Source: CAD feature listing. Evaluate the final solid. Frame: model axes, mm. A direction names the side the tool comes from. Give positions to 0.01 mm unless a question says otherwise; leave off trailing zeros. Order: outer loops, then holes, each group sorted by start corner. A loop starts at its lowest first (then second) coordinate and runs counter-clockwise, first axis right, second up.
Autodesk Inventor part; units mm, degrees
ref_plane "YZ Plane" through (0, 0, 0) normal (1, 0, 0) x (0, 1, 0)
ref_plane "XZ Plane" through (0, 0, 0) normal (0, 1, 0) x (-1, 0, 0)
ref_plane "XY Plane" through (0, 0, 0) normal (0, 0, 1) x (1, 0, 0)
sketch "Sketch1" plane through (0, 0, 0) normal (0, 1, 0) x (-1, 0, 0)
  line L0 (0, 0) -> (-120, 0)
  line L1 (-120, 0) -> (-120, -100)
  line L2 (-120, -100) -> (0, -100)
  line L3 (0, -100) -> (0, 0)
  dimension "d0" = 120
  dimension "d1" = 100
extrude "Extrusion1" add sketch "Sketch1" along normal blind 3
sketch "Sketch2" plane through (0, 3, 0) normal (0, 1, 0) x (1, 0, 0)
  line L0 (0, 100) -> (0, 0) construction
  line L1 (0, 0) -> (3, 0) construction
  line L2 (3, 0) -> (3, 3) construction
  line L3 (3, 3) -> (0, 3) construction
  line L4 (0, 3) -> (0, 0) construction
  line L5 (120, 100) -> (0, 100) construction
  line L6 (120, 100) -> (117, 100) construction
  line L7 (117, 100) -> (117, 97) construction
  line L8 (117, 97) -> (120, 97) construction
  line L9 (120, 97) -> (120, 100) construction
  line L10 (3, 3) -> (117, 3)
  line L11 (117, 3) -> (117, 97)
  line L12 (117, 97) -> (3, 97)
  line L13 (3, 97) -> (3, 3)
  line L14 (120, 0) -> (120, 100)
  line L15 (0, 0) -> (120, 0)
  line L16 (120, 0) -> (120, 100)
  line L17 (120, 100) -> (0, 100)
  line L18 (0, 100) -> (0, 0)
  dimension "d4" = 3
  dimension "d5" = 3
  dimension "d6" = 3
  dimension "d7" = 3
extrude "Extrusion2" add sketch "Sketch2" along normal blind 97
ref_plane "Work Plane1" through (155, 0, 0) normal (1, 0, 0) x (0, 0, -1)
sketch "Sketch3" plane through (155, 0, 0) normal (1, 0, 0) x (0, 0, -1)
  line L0 (0, 0) -> (0, 100) construction
  line L1 (0, 0) -> (50, 0) construction
  line L2 (100, 0) -> (0, 0) construction
  line L3 (50, 0) -> (50, 35) construction
  line L4 (50, 35) -> (43, 35) construction
  line L5 (50, 35) -> (50, 73) construction
  line L6 (50, 73) -> (40, 73) construction
  line L7 (40, 73) -> (40, 54) construction
  line L8 (43, 35) -> (40, 54)
  line L9 (40, 54) -> (40, 73)
  line L10 (3, 100) -> (97, 100) construction
  line L11 (50, 100) -> (15, 100) construction
  line L12 (15, 100) -> (15, 97)
  line L13 (15, 97) -> (40, 73)
  line L14 (15, 100) -> (43, 73)
  line L15 (43, 73) -> (43, 54)
  line L16 (43, 35) -> (45, 35)
  line L17 (43, 54) -> (45, 35)
  dimension "d11" = 35
  dimension "d12" = 7
  dimension "d13" = 38
  dimension "d14" = 10
  dimension "d15" = 35
  dimension "d16" = 3
  dimension "d81" = 19
  dimension "d82" = 3
  dimension "d83" = 2
  dimension "d84" = 19
revolve "Revolution1" add sketch "Sketch3" angle 360 about axis through (155, 35, -50) along (0, 1, 0)
sketch "Sketch4" plane through (0, 100, 0) normal (0, 1, 0) x (1, 0, 0)
  line L0 (120, 0) -> (120, 100)
  line L1 (120, 0) -> (120, 3)
  line L2 (120, 100) -> (0, 100)
  line L3 (120, 100) -> (120, 97)
  line L4 (120, 97) -> (120, 3)
  circle A0 centre (155, 50) radius 5
  circle A1 centre (155, 50) radius 35
  circle A2 centre (155, 50) radius 38
  line L5 (120, 0) -> (120, 100)
  line L6 (120, 0) -> (155, 12)
  line L7 (155, 88) -> (120, 100)
  point P0 (0, 0)
  point P1 (120, 50)
  dimension "d18" = 3
  dimension "d19" = 3
  dimension "d89" = 70
  dimension "d90" = 3
extrude "Extrusion3" add sketch "Sketch4" against normal blind 3 contours L0 A2 L6 | A2 L0 | L0 L7 A2 picked at (191.3899, 55.4147)
sketch "Sketch5" plane through (0, 100, 0) normal (0, 1, 0) x (1, 0, 0)
  line L0 (120, 0) -> (120, 100)
  line L1 (0, 100) -> (0, 0)
  line L2 (120, 0) -> (0, 0)
  line L3 (0, 0) -> (0, 100)
  line L4 (0, 100) -> (120, 100)
  line L5 (120, 100) -> (120, 0)
  circle A0 centre (155, 50) radius 35
  line L6 (117, 3) -> (117, 97)
  line L7 (117, 3) -> (3, 3)
  line L8 (3, 3) -> (3, 97)
  line L9 (117, 3) -> (3, 3)
  line L10 (3, 3) -> (3, 97)
  line L11 (3, 97) -> (117, 97)
  line L12 (117, 97) -> (117, 3)
  circle A1 centre (155, 50) radius 35
  circle A2 centre (155, 50) radius 38
  line L13 (0, 0) -> (120, 0)
  line L14 (120, 100) -> (155, 88)
  line L15 (120, 100) -> (155, 88)
  line L16 (155, 12) -> (120, 0)
  line L17 (120, 0) -> (155, 12)
  line L18 (120, 50) -> (120, 0)
  line L19 (120, 3) -> (155, 15)
  line L20 (120, 100) -> (120, 50)
  line L21 (120, 97) -> (155, 85)
  line L22 (155, 88) -> (120, 100)
  line L23 (117, 3) -> (120, 3)
  line L24 (120, 97) -> (117, 97)
  dimension "d85" = 3
  dimension "d91" = 37
  dimension "d92" = 37
extrude "Extrusion4" add sketch "Sketch5" along normal blind 10 contours L2 L1 L4 L0 L24 L11 L8 L7 L23 | L0 L19 A2 L16 | A2 L19 A0 L21 | L14 A2 L21 L0
ref_plane "Work Plane2" through (3, 3, -65) normal (0, 0, 1) x (1, 0, 0)
sketch "Sketch6" plane through (3, 3, -65) normal (0, 0, 1) x (1, 0, 0)
  line L0 (0, 0) -> (0, 107)
  line L1 (0, 0) -> (0, 21.21)
  line L2 (0, 0) -> (114, 0)
  line L3 (0, 0) -> (21.21, 0)
  line L4 (114, 0) -> (0, 0)
  line L5 (0, 21.21) -> (21.21, 0)
  line L6 (0, 21.21) -> (0, 17.21)
  line L7 (0, 17.21) -> (17.21, 0)
  point P0 (-3, -3)
  point P1 (0, 17.21)
  point P2 (17.21, 0)
  point P3 (21.21, 0)
  point P4 (0, 97)
  dimension "d26" = 21.21
  dimension "d27" = 21.21
  dimension "d28" = 4
extrude "Extrusion5" add sketch "Sketch6" along normal blind 30 contours L0 L5 L2 L7
sketch "Sketch7" plane through (3, 24.21, -65) normal (0.7071, 0.7071, 0) x (-0.7071, 0.7071, 0)
  line L0 (-29.9955, 30) -> (0, 30)
  line L1 (-14.9977, 30) -> (-14.9977, 15)
  circle A0 centre (-14.9977, 15) radius 11.5
  point P0 (-14.9977, 65)
  dimension "d31" = 15
  dimension "d32" = 23
extrude "Extrusion6" cut sketch "Sketch7" against normal blind 3.6
sketch "Sketch11" plane through (3, 3, -65) normal (0, 0, 1) x (1, 0, 0)
  line L0 (18.7367, 2.4733) -> (16.7367, 0.4733) construction
  line L1 (18.7367, 2.4733) -> (148.7367, 132.4733) construction
  line L2 (2.4733, 18.7367) -> (0.4733, 16.7367) construction
  line L3 (2.4733, 18.7367) -> (132.4733, 148.7367) construction
  line L4 (113.7569, 97.4935) -> (95.3721, 115.8782) construction
  line L5 (95.3721, 115.8782) -> (92.3721, 112.8782) construction
  line L6 (92.3721, 112.8782) -> (113.7569, 91.4935) construction
  line L7 (117, 97) -> (145, 70)
  line L8 (117, 97) -> (113.4034, 97.847)
  line L9 (113.4034, 97.847) -> (95.3721, 115.8782)
  line L10 (95.3721, 115.8782) -> (92.3721, 112.8782)
  line L11 (92.3721, 112.8782) -> (110.7569, 94.4935)
  line L12 (110.7569, 94.4935) -> (114, 85.7766)
  line L13 (114, 0) -> (114, 97)
  line L14 (114, 85.7766) -> (117, 85.7766)
  line L15 (117, 85.7766) -> (117, 97)
  line L16 (117, 94) -> (117, 107)
  point P0 (-3, -3)
  dimension "d65" = 130
  dimension "d66" = 130
  dimension "d67" = 26
  dimension "d68" = 3
  dimension "d69" = 134.3788
  dimension "d70" = 4.2426
  dimension "d71" = 49.4689
  dimension "d72" = 49.4689
  dimension "d73" = 25.634
  dimension "d74" = 149.293
  dimension "d75" = 0
extrude "Extrusion8" add sketch "Sketch11" along normal blind 30
sketch "Sketch12" plane through (3, 24.21, -65) normal (0.7071, 0.7071, 0) x (-0.7071, 0.7071, 0)
  line L0 (-14.9977, -32) -> (-14.9977, 62)
  circle A0 centre (-14.9977, 15) radius 11.5
  point P0 (-14.9977, 65)
  dimension "d78" = 23
extrude "Extrusion9" cut sketch "Sketch12" along normal through all
properties part number "Resoar V2"
1) First-contact query: pin 1 Ø4 at (y, z) = (81, -59.5) entering from -X; pin 2 Ø4 at (x, z) = (140, -85.5) entering from -Y; pin 3 Ø10 at (x, y) = (148.5, 94) entering from -Z; pin 4 Ø6 at (y, z) = (44, -75.5) entering from +X. Flat tips, straight axial feed; report the tip coordinate or a pass-through.
Checks:
pin 1: stops at x = 0
pin 2: stops at y = 97
pin 3: stops at z = -91.6
pin 4: stops at x = 120
2) Section query D-D on y = 108. State how many separate pieces and enclosed holes the cut face has, and give its area (3 significant figures).
Checks:
separate pieces: 3
enclosed holes: 1
area: 1,600 mm2
3) Reachability of faces 1 (the face through (0, 54, -51)), 2 (the face through (108, 106, -65)), 3 (the face through (115.356, 93.196, -50.21)), 4 (the face through (120, 48, -49)) from +Z, -Z, +X, -X, +Y, -Y: full face, straight path, thin tool, end or side. Return the list, or none.
Checks:
face 1: +Z, -Z, -X, +Y, -Y
face 2: +Y
face 3: none
face 4: +Z, -Z, -Y
4) Section query B-B on x = 91.5. Output: boundary loops of the cut face in (y, z).
Checks:
outline: (0, -100) - (110, -100) - (110, -97) - (3, -97) - (3, -3) - (110, -3) - (110, 0) - (0, 0) - close
5) Section query C-C on y = 93.5. Output: boundary loops of the cut face in (x, z), and give its area (3 significant figures).
Checks:
outline: (0, -100) - (120, -100) - (120, 0) - (0, 0) - close; circle Ø62.71 at (155, -50); hole (3, -97) - (117, -97) - (117, -65) - (115.24, -65) - (115.24, -35) - (117, -35) - (117, -3) - (3, -3) - close; hole circle Ø56.52 at (155, -50)
area: 1,920 mm2
6) Ray query, L1, parallel to X at y = 14.5, z = -30.5; L2, parallel to Z at x = 98.5, y = 22.5; L3, parallel to X at y = 59, z = -50. Return the intervals inside material, ascending.
Checks:
L1: x = 0 to 3, 117 to 120
L2: z = -100 to -97, -3 to 0
L3: x = 0 to 3, 117 to 120, 145 to 148, 162 to 165
7) Pull-direction query (Y, two-part tool) for faces 5 (the face through (192.99, 103.59, -49.16)), 6 (the face through (3.84, 19.37, -56.88)), 7 (the face through (121, 97, -61)); classes: +Y half, -Y half, draft (parallel to the pull), parting line (faces both ways), or undercut.
Checks:
face 5: draft
face 6: undercut
face 7: -Y half
8) Section query A-A on y = 39. Output: boundary loops of the cut face in (x, z).
Checks:
outline: (0, -100) - (120, -100) - (120, 0) - (0, 0) - close; circle Ø15.26 at (155, -50); hole (3, -97) - (117, -97) - (117, -3) - (3, -3) - close; hole circle Ø10.84 at (155, -50)
